Job drawing, mm, ordinate dimensions from the low corner. One solid piece. Round coordinates to 2 decimals unless told otherwise and drop trailing zeros. Order: outer loops, then holes, each group sorted by start corner. A loop starts at its lowest first (then second) coordinate and runs counter-clockwise, first axis right, second up. Notation, with made-up numbers: (34, 14.25) -> (78, 14.25) arc R24 ccw to (78, 45.25) -> close; hole circle Ø11 at (35, 11). An arc over 180 degrees is marked (long way). Write item = value, one per line.
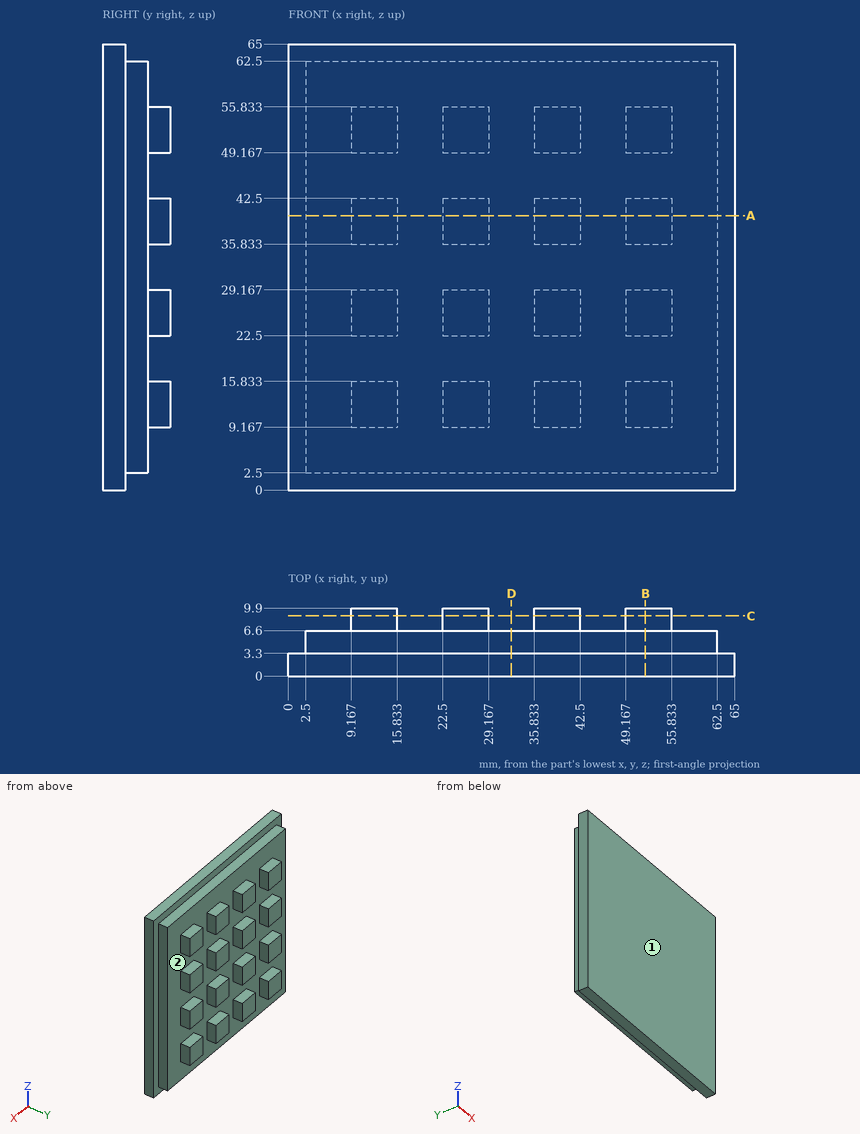
Q1. Mould opens along Z. For the marked faces 1 and 2 say: released by +Z, released by -Z, zero draft, split by the parting line, or undercut.
Check values:
face_1 = zero draft
face_2 = undercut
Q2. Cut at C-C, the plane y = 8.75. Give the number of separate pieces and of enclosed holes in the cut face, and give its area (3 significant figures).
Check values:
separate_pieces = 16
enclosed_holes = 0
area = 711 mm²
Q3. Cut at D-D, the plane x = 32.5. List the corners of the cut face in (y, z).
Check values:
outline = (0, 0) -> (3.3, 0) -> (3.3, 2.5) -> (6.6, 2.5) -> (6.6, 62.5) -> (3.3, 62.5) -> (3.3, 65) -> (0, 65) -> close
Q4. Flat gauge pins, fed straight in: pin 1 (1 mm diameter, centred on x = 38, y = 9, fed in from +Z); pin 2 (1 mm diameter, centred on x = 24.5, y = 7.5, fed in from -Z); pin 3 (1.6 mm diameter, centred on y = 7.5, z = 53, fed in from +X); pin 4 (4 mm diameter, centred on x = 23, y = 3.5, fed in from +Z). Where does each tip first touch, or does it go through?
Check values:
pin_1 = 55.83
pin_2 = 9.17
pin_3 = 55.83
pin_4 = 65
Q5. Probe probe 1 along X at (y, z) = (6.75, 15.5); probe 2 along X at (y, z) = (3.5, 12). List the from-to ranges inside material, lowest first.
Check values:
probe_1 = 9.17 to 15.83, 22.5 to 29.17, 35.83 to 42.5, 49.17 to 55.83
probe_2 = 2.5 to 62.5
Q6. Cut at A-A, the plane z = 40. List the corners of the cut face in (x, y).
Check values:
outline = (0, 0) -> (65, 0) -> (65, 3.3) -> (62.5, 3.3) -> (62.5, 6.6) -> (55.83, 6.6) -> (55.83, 9.9) -> (49.17, 9.9) -> (49.17, 6.6) -> (42.5, 6.6) -> (42.5, 9.9) -> (35.83, 9.9) -> (35.83, 6.6) -> (29.17, 6.6) -> (29.17, 9.9) -> (22.5, 9.9) -> (22.5, 6.6) -> (15.83, 6.6) -> (15.83, 9.9) -> (9.17, 9.9) -> (9.17, 6.6) -> (2.5, 6.6) -> (2.5, 3.3) -> (0, 3.3) -> close
Q7. Cut at B-B, the plane x = 52. List the corners of the cut face in (y, z).
Check values:
outline = (0, 0) -> (3.3, 0) -> (3.3, 2.5) -> (6.6, 2.5) -> (6.6, 9.17) -> (9.9, 9.17) -> (9.9, 15.83) -> (6.6, 15.83) -> (6.6, 22.5) -> (9.9, 22.5) -> (9.9, 29.17) -> (6.6, 29.17) -> (6.6, 35.83) -> (9.9, 35.83) -> (9.9, 42.5) -> (6.6, 42.5) -> (6.6, 49.17) -> (9.9, 49.17) -> (9.9, 55.83) -> (6.6, 55.83) -> (6.6, 62.5) -> (3.3, 62.5) -> (3.3, 65) -> (0, 65) -> close
